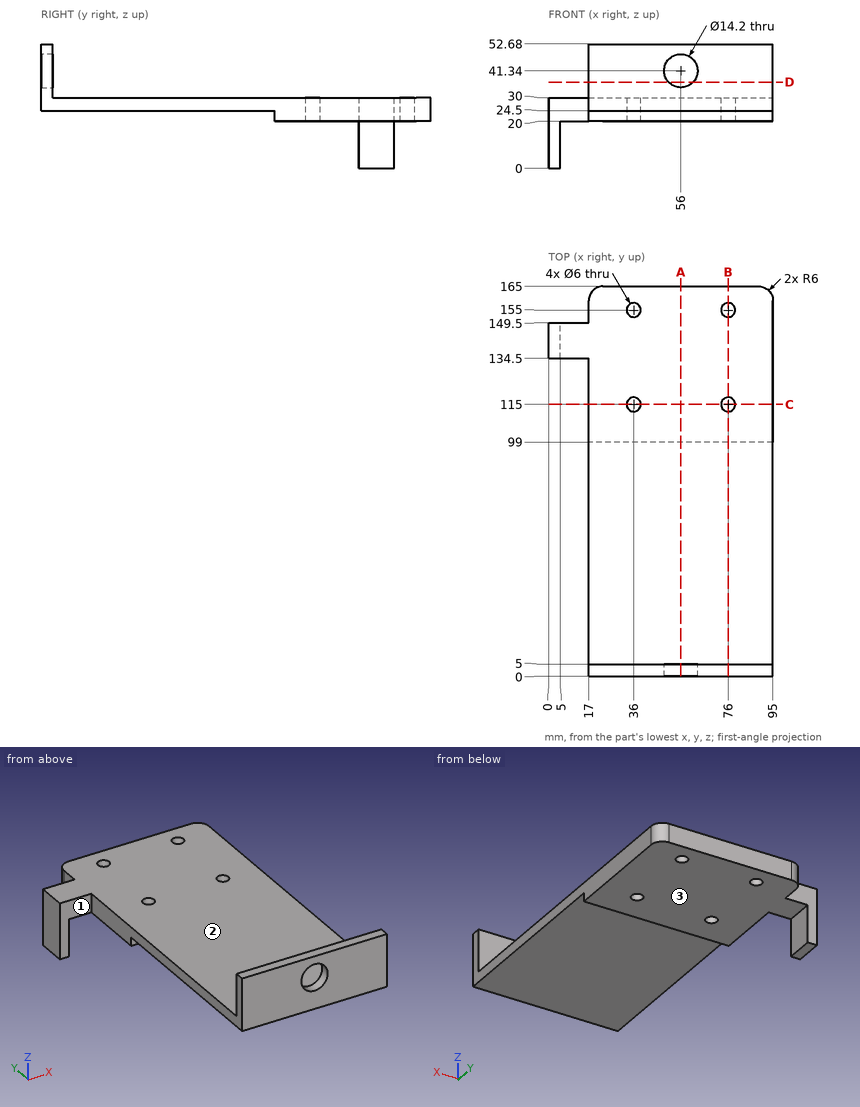
For this review, use the dimensioned drawing (mm, ordinates from the lowest corner) and the shaded views. A direction names the side the tool comes from. Coordinates: 2 decimals unless noted, no trailing zeros. Loops run counter-clockwise (first coordinate to the right, second up) from the corner with the lowest first, then second, coordinate; pieces in that order, holes last.
1. Add section D-D, the plane z = 36.5. Give the boundary of the cut face in (x, y).
2. Add section B-B, the plane x = 76. Give the boundary of the cut face in (y, z), then the cut area to 3 significant figures.
3. For line 1 (Y direction, x = 36, z = 24); line 2 (X direction, y = 155, z = 24.5); line 3 (Y direction, x = 76, z = 25), list the stretches that pass through material, from the lowest coordinate up.
4. Insertion check: P1, Ø8.5, axis at x = 10.5, z = 16, coming from the -Y side; P2, Ø4, axis at x = 36.5, y = 47, coming from the +Z side; P3, Ø3, axis at y = 153.5, z = 26.5, coming from the -X side. Each pin has a flat end and moves straight along its axis. Give the tip position at first contact, or say it passes through.
5. Add section C-C, the plane y = 115. Give the boundary of the cut face in (x, z).
6. Add section A-A, the plane x = 56. Give the boundary of the cut face in (y, z).
7. For the marked faces 1, 2 and 3, list the 3-axis set-ups (+Z, -Z, +X, -X, +Y, -Y) from which the entire face can be reached by the end or side of a thin tool; tool diameter is ignored.
Result:
1. outline: (17, 0) - (50.81, 0) - (50.81, 5) - (17, 5) - close; (61.19, 0) - (95, 0) - (95, 5) - (61.19, 5) - close
2. outline: (0, 24.5) - (99, 24.5) - (99, 20) - (112, 20) - (112, 30) - (5, 30) - (5, 52.68) - (0, 52.68) - close; (118, 20) - (152, 20) - (152, 30) - (118, 30) - close; (158, 20) - (165, 20) - (165, 30) - (158, 30) - close
2. area: 1,200 mm2
3. line 1: y = 99 to 112, 118 to 152, 158 to 165
3. line 2: x = 17 to 33, 39 to 73, 79 to 95
3. line 3: y = 0 to 112, 118 to 152, 158 to 165
4. P1: stops at y = 134.5
4. P2: stops at z = 30
4. P3: stops at x = 17
5. outline: (17, 20) - (33, 20) - (33, 30) - (17, 30) - close; (39, 20) - (73, 20) - (73, 30) - (39, 30) - close; (79, 20) - (95, 20) - (95, 30) - (79, 30) - close
6. outline: (0, 24.5) - (99, 24.5) - (99, 20) - (165, 20) - (165, 30) - (5, 30) - (5, 34.24) - (0, 34.24) - close; (0, 48.44) - (5, 48.44) - (5, 52.68) - (0, 52.68) - close
7. face 1: +Z, -Z, -X, -Y
7. face 2: +Z, +X, -X, +Y
7. face 3: -Z, +X, +Y, -Y
